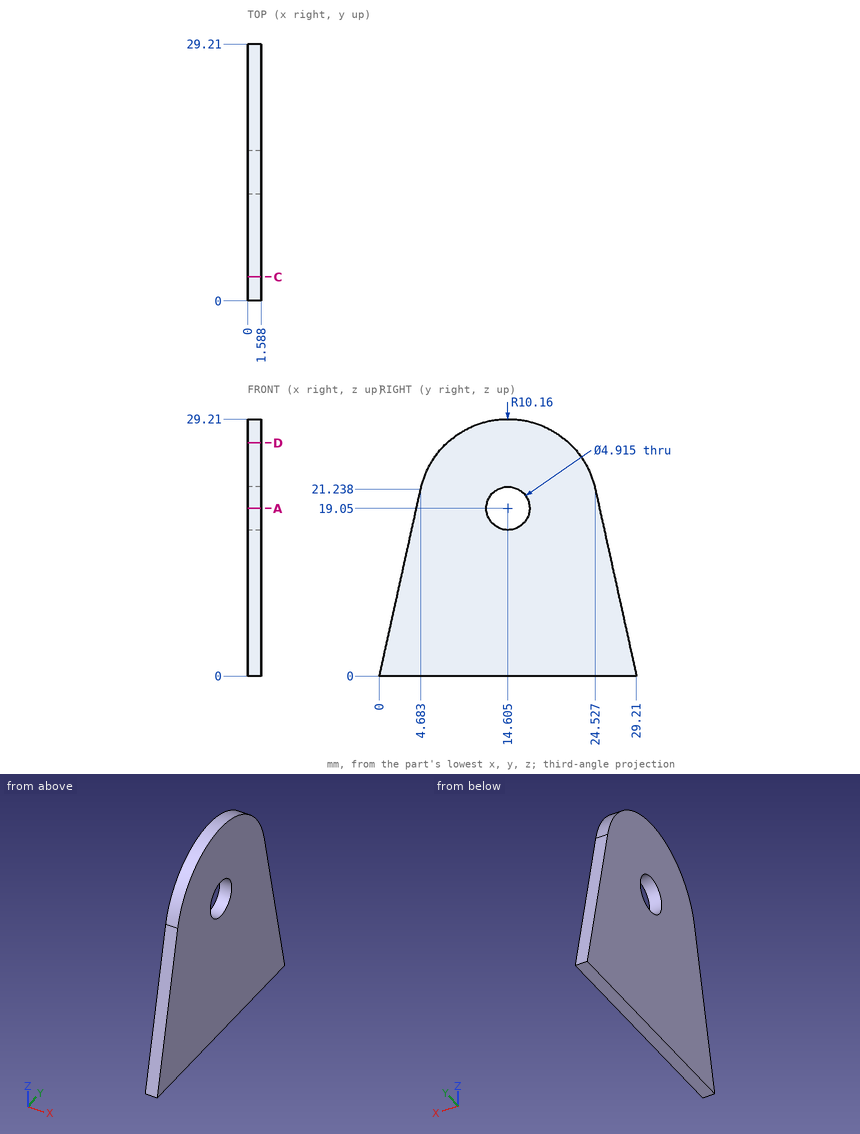
Check sheet for the drawn part. Datum: minimum x, y, z corner. Units: mm. Give positions to 0.01 mm unless a question says otherwise; leave off trailing zeros. Order: outer loops, then holes, each group sorted by start corner. A loop starts at its lowest first (then second) coordinate and runs counter-clockwise, first axis right, second up. Notation, with made-up numbers: (54.25, -1.75) - (64.25, -1.75) arc R30 cw to (64.25, 22.25) - close; hole circle Ø2 at (-37.5, 71). An arc over 180 degrees is marked (long way). Answer as a JSON object with one key per item and string values.
(1) Cross-section at D-D (z = 26.5). Record the cut outline in (x, y).
Report:
{"outline": "(0, 7.7) - (1.59, 7.7) - (1.59, 21.51) - (0, 21.51) - close"}
(2) Cross-section at C-C (y = 2.75). Record the cut outline in (x, z), then the cut area to 3 significant figures.
Report:
{"outline": "(0, 0) - (1.59, 0) - (1.59, 12.47) - (0, 12.47) - close", "area": "19.8 mm^2"}
(3) Material ranges on line 1 (Z direction, x = 0.5, y = 15.25); line 2 (Y direction, x = 0.15, z = 20.5); line 3 (Y direction, x = 1.25, z = 19.05), recorded low to high.
Report:
{"line 1": "0 to 16.68, 21.42 to 29.19", "line 2": "4.52 to 12.62, 16.59 to 24.69", "line 3": "4.2 to 12.15, 17.06 to 25.01"}
(4) Cross-section at A-A (z = 19.05). Record the cut outline in (x, y).
Report:
{"outline": "(0, 4.2) - (1.59, 4.2) - (1.59, 12.15) - (0, 12.15) - close; (0, 17.06) - (1.59, 17.06) - (1.59, 25.01) - (0, 25.01) - close"}
